from build123d import *

# Parameters (mm, degrees)
CROQUIS1_R              = 5.125
SALIENTE_EXTRUIR1_DEPTH = 6.35


with BuildPart() as part:
    # Croquis1 → Saliente-Extruir1 (new, symmetric)
    with BuildSketch(Plane.XY):
        with BuildLine():
            Line((-37.5, 68), (37.5, 68))
            ThreePointArc((37.5, 68), (41.035533906, 66.535533906), (42.5, 63))
            Line((42.5, 63), (42.5, -63))
            ThreePointArc((42.5, -63), (41.035533906, -66.535533906), (37.5, -68))
            Line((37.5, -68), (-37.5, -68))
            ThreePointArc((-37.5, -68), (-41.035533906, -66.535533906), (-42.5, -63))
            Line((-42.5, -63), (-42.5, 63))
            ThreePointArc((-42.5, 63), (-41.035533906, 66.535533906), (-37.5, 68))
        make_face()
        with Locations((-27.5, 55)):
            Circle(CROQUIS1_R, mode=Mode.SUBTRACT)
        with Locations(Location((27.5, 55, 0), (0, 0, 180))):
            Circle(CROQUIS1_R, mode=Mode.SUBTRACT)
        with Locations((0, -55)):
            Circle(CROQUIS1_R, mode=Mode.SUBTRACT)
        with Locations((0, -25)):
            Circle(CROQUIS1_R, mode=Mode.SUBTRACT)
    extrude(amount=SALIENTE_EXTRUIR1_DEPTH, both=True)


solid = part.part
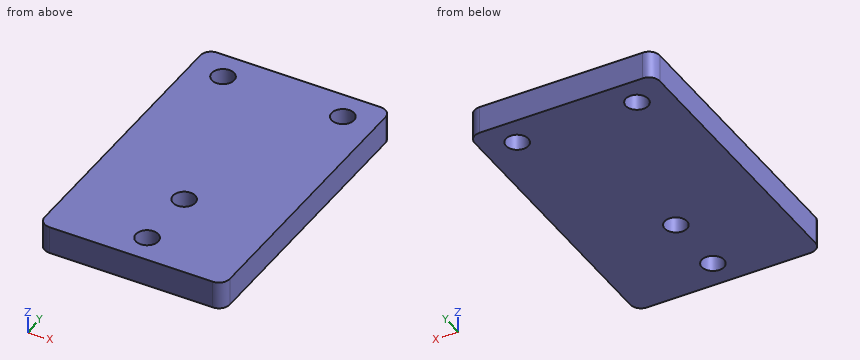
Read the model definition and answer for the solid it produces. Units are mm, in the model's axes. Give positions to 0.01 mm unless a question says otherwise; leave off trailing zeros. Write each loop counter-clockwise with the first axis right and the second up, starting at its lowest first coordinate (ties: lowest second). Pieces come first, ordered by that corner, then holes. Notation, with made-up numbers: (-15.75, 27) - (27.25, 27) arc R17 cw to (27.25, 57) - close; hole circle Ø4 at (33.5, 38.5). An arc over 180 degrees is marked (long way). Use CSV: the item, a comma, the result in double quotes. Start each with the question number.
Item 1: The part is cut by section C-C, the plane z = 2.5. Give the vertices of the cut face in (x, y) (3 decimals), and give its area (3 significant figures).
Item 2: A flat-ended cylindrical pin translates along its axis: P1, Ø8, axis at x = 27.5, y = 55, coming from the +Z side. Find the tip coordinate at first contact, or state that the pin passes through.
Item 3: The part is cut by section D-D, the plane y = -25. Give the vertices of the cut face in (x, z) (3 decimals), and give its area (3 significant figures).
Item 4: The part is cut by section A-A, the plane x = -27.5. Give the vertices of the cut face in (y, z) (3 decimals).
Item 5: Consider line 1 (Y direction, x = 0, z = -1.25) (3 decimals); line 2 (Y direction, x = 27.5, z = -0.75) (3 decimals); line 3 (Y direction, x = 4, z = 0). Determine where each line is inside the solid, lowest interval first.
Item 6: The part is cut by section B-B, the plane y = 55. Give the vertices of the cut face in (x, z) (3 decimals), and give its area (3 significant figures).
Taken from the geometry:
1,outline,"(-42.5, -63) arc R5 ccw to (-37.5, -68) - (37.5, -68) arc R5 ccw to (42.5, -63) - (42.5, 63) arc R5 ccw to (37.5, 68) - (-37.5, 68) arc R5 ccw to (-42.5, 63) - close; hole circle Ø10.25 at (-27.5, 55); hole circle Ø10.25 at (0, -55); hole circle Ø10.25 at (0, -25); hole circle Ø10.25 at (27.5, 55)"
1,area,"11,200 mm2"
2,P1,"through"
3,outline,"(-42.5, -6.35) - (-5.125, -6.35) - (-5.125, 6.35) - (-42.5, 6.35) - close; (5.125, -6.35) - (42.5, -6.35) - (42.5, 6.35) - (5.125, 6.35) - close"
3,area,"949 mm2"
4,outline,"(-68, -6.35) - (49.875, -6.35) - (49.875, 6.35) - (-68, 6.35) - close; (60.125, -6.35) - (68, -6.35) - (68, 6.35) - (60.125, 6.35) - close"
5,line 1,"-68 to -60.125, -49.875 to -30.125, -19.875 to 68"
5,line 2,"-68 to 49.875, 60.125 to 68"
5,line 3,"-68 to -58.2, -51.8 to -28.2, -21.8 to 68"
6,outline,"(-42.5, -6.35) - (-32.625, -6.35) - (-32.625, 6.35) - (-42.5, 6.35) - close; (-22.375, -6.35) - (22.375, -6.35) - (22.375, 6.35) - (-22.375, 6.35) - close; (32.625, -6.35) - (42.5, -6.35) - (42.5, 6.35) - (32.625, 6.35) - close"
6,area,"819 mm2"
